Design review of the part shown in the three views and the two pictorial views. Dimensions are in mm from the part's minimum x, y and z. A direction names the side the tool comes from. Round coordinates to 2 decimals unless told otherwise and drop trailing zeros. Loops run counter-clockwise (first coordinate to the right, second up) from the corner with the lowest first, then second, coordinate; pieces in that order, holes last.
1. Clearance check with flat-ended pins moving along their axes: pin 1 Ø1.5 at (x, z) = (9.5, 2.5) entering from +Y (1 decimal); pin 2 Ø5 at (x, z) = (11, 7.5) entering from +Y (1 decimal); pin 3 Ø1.5 at (x, y) = (6.5, 8.5) entering from +Z (1 decimal). State where each tip first meets the part, or that it passes through.
2. Tool access review of the marked faces 1 and 2: name each direction out of +Z, -Z, +X, -X, +Y, -Y from which nothing blocks a thin tool from reaching the whole face with its end or side.
3. Consider section D-D on x = 1. State the section outline as (y, z) points.
4. Consider section C-C on x = 8.5. State the section outline as (y, z) points (1 decimal).
5. Consider section A-A on z = 8.75. State the section outline as (x, y) points, then the cut area to 3 significant figures.
6. To check wall thickness, follow line 1 along Z through (x, y) = (9, 5.5) (1 decimal); line 2 along X through (y, z) = (9.75, 2.5); line 3 along Z through (x, y) = (8, 7.25) (1 decimal). State the ranges of each line that lie inside material, in increasing order.
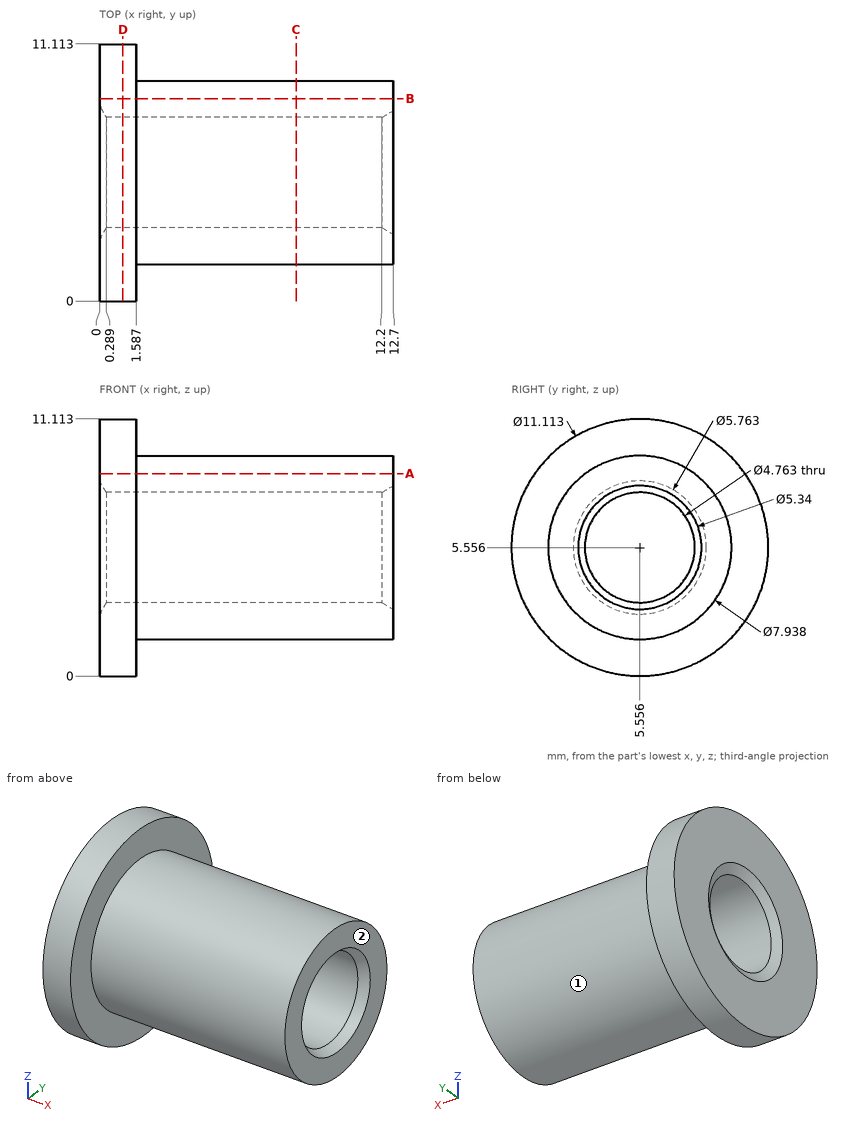
Resolved:
1. pin 1: stops at y = 8.8
1. pin 2: stops at y = 9.5
1. pin 3: stops at z = 8.9
2. face 1: +X
2. face 2: +Z, -Z, +X, +Y, -Y
3. outline: circle Ø11.11 at (5.56, 5.56); hole circle Ø4.76 at (5.56, 5.56)
4. outline: circle Ø7.9 at (5.6, 5.6); hole circle Ø4.8 at (5.6, 5.6)
5. outline: (0, 1.01) - (1.59, 1.01) - (1.59, 3.2) - (12.7, 3.2) - (12.7, 7.91) - (1.59, 7.91) - (1.59, 10.1) - (0, 10.1) - close
5. area: 66.8 mm2
6. line 1: z = 1.6 to 3.2, 7.9 to 9.5
6. line 2: x = 0 to 1.59
6. line 3: z = 2 to 3.9, 7.2 to 9.1
